Check sheet for the modelled part. Datum: model origin and axes. Units: mm. A direction names the side the tool comes from. Give positions to 0.01 mm unless a question says otherwise; leave off trailing zeros. Order: outer loops, then holes, each group sorted by start corner. A loop starts at its lowest first (then second) coordinate and runs counter-clockwise, first axis right, second up.
```python
from build123d import *

# Parameters (mm, degrees)
CROQUIS1_R              = 5.3
CROQUIS1_R_2            = 1.511434147
SALIENTE_EXTRUIR1_DEPTH = 3
CROQUIS3_R              = 1.8
CROQUIS3_R_2            = 5.3
SALIENTE_EXTRUIR2_DEPTH = 3


with BuildPart() as part:
    # Croquis1 → Saliente-Extruir1 (new body)
    with BuildSketch(Plane(origin=(0, 0, 0), x_dir=(1, 0, 0), z_dir=(0, 1, 0))):
        with BuildLine():
            Line((10.649291245, -23.45570863), (10.649291245, 1.133383189))
            ThreePointArc((10.649291245, 1.133383189), (-1.350708755, 19.76429137), (-13.350708755, 1.133383189))
            Line((-13.350708755, 1.133383189), (-13.350708755, -23.45570863))
            Line((-13.350708755, -23.45570863), (10.649291245, -23.45570863))
        make_face()
        with Locations((-1.350708755, 6.58429137)):
            Circle(CROQUIS1_R, mode=Mode.SUBTRACT)
        with Locations((6.073912448, 14.008912573)):
            Circle(CROQUIS1_R_2, mode=Mode.SUBTRACT)
        with Locations((6.073912448, -0.840329832)):
            Circle(CROQUIS1_R_2, mode=Mode.SUBTRACT)
        with Locations((-8.775329957, -0.840329832)):
            Circle(CROQUIS1_R_2, mode=Mode.SUBTRACT)
        with Locations((-8.775329957, 14.008912573)):
            Circle(CROQUIS1_R_2, mode=Mode.SUBTRACT)
    extrude(amount=SALIENTE_EXTRUIR1_DEPTH)

    # Croquis3 → Saliente-Extruir2 (add)
    with BuildSketch(Plane.XY.offset(23.45570863)):
        with BuildLine():
            Line((10.649291245, 3), (-13.350708755, 3))
            Line((-13.350708755, 3), (-13.350708755, -22.057235679))
            ThreePointArc((-13.350708755, -22.057235679), (-1.494791792, -40.779605827), (10.649291245, -22.242854272))
            Line((10.649291245, -22.242854272), (10.649291245, 3))
        make_face()
        with Locations((-8.817480498, -35.024621202)):
            Circle(CROQUIS3_R, mode=Mode.SUBTRACT)
        with Locations((-8.817480498, -20.175378798)):
            Circle(CROQUIS3_R, mode=Mode.SUBTRACT)
        with Locations((6.031761906, -20.175378798)):
            Circle(CROQUIS3_R, mode=Mode.SUBTRACT)
        with Locations((6.031761906, -35.024621202)):
            Circle(CROQUIS3_R, mode=Mode.SUBTRACT)
        with Locations((-1.392859296, -27.6)):
            Circle(CROQUIS3_R_2, mode=Mode.SUBTRACT)
    extrude(amount=SALIENTE_EXTRUIR2_DEPTH)


solid = part.part
```
Q1. Tool access check on faces 1 (the flat face through (-2, 0, 2)), 2 (the flat face through (-2, -19, 26.456)), 3 (the flat face through (10.649, 1, 18)). Record the directions out of +Z, -Z, +X, -X, +Y, -Y that give a thin tool (end or side, any length) a straight path to the whole face; none if there is none.
Q2. Sectioned sample at D-D, the plane z = -9. Record the cut outline in (x, y), plus the area to 3 significant figures.
Q3. Sectioned sample at C-C, the plane x = -9.25. Record the cut outline in (y, z).
Q4. Material ranges on line 1 (Y direction, x = 4.5, z = 20.5); line 2 (Z direction, x = 3.25, y = -35), recorded low to high.
Q5. Sectioned sample at A-A, the plane y = -27.6. Record the cut outline in (x, z), plus the area to 3 significant figures.
Q6. Sectioned sample at B-B, the plane x = -4.5. Record the cut outline in (y, z), plus the area to 3 significant figures.
Q7. Draft check along X on faces 4 (the flat face through (-13.351, 1, 19)), 5 (the flat face through (-2, -20, 23.456)), 6 (the cylindrical face through (1.5, 1.48, -11.05)). Enter one of: pulls with the +X half, pulls with the -X half, needs draft (parallel to the pull), parting line crosses it, or undercut.
Q8. Go/stop test with flat-tipped pins: P1, Ø8, axis at x = 5, y = -22.5, coming from the -Z side; P2, Ø13, axis at x = -0.5, z = -2.5, coming from the -Y side. Record where each tip stops, or that it passes through.
Filled in:
1. face 1: -Z, +X, -X, -Y
1. face 2: +Z, +X, -X, +Y, -Y
1. face 3: +Z, +X, +Y
2. outline: (-14.31, 0) - (-6.07, 0) - (-6.07, 3) - (-14.31, 3) - close; (3.37, 0) - (11.61, 0) - (11.61, 3) - (3.37, 3) - close
2. area: 49.4 mm2
3. outline: (-38.18, 23.46) - (-36.77, 23.46) - (-36.77, 26.46) - (-38.18, 26.46) - close; (-33.28, 23.46) - (-21.92, 23.46) - (-21.92, 26.46) - (-33.28, 26.46) - close; (-18.43, 23.46) - (0, 23.46) - (0, 2.28) - (3, 2.28) - (3, 26.46) - (-18.43, 26.46) - close; (0, -17.13) - (3, -17.13) - (3, -15.44) - (0, -15.44) - close; (0, -12.57) - (3, -12.57) - (3, -0.59) - (0, -0.59) - close
4. line 1: y = 0 to 3
4. line 2: z = 23.46 to 26.46
5. outline: (-14.57, 23.46) - (-6.69, 23.46) - (-6.69, 26.46) - (-14.57, 26.46) - close; (3.91, 23.46) - (11.79, 23.46) - (11.79, 26.46) - (3.91, 26.46) - close
5. area: 47.3 mm2
6. outline: (-40.41, 23.46) - (-31.89, 23.46) - (-31.89, 26.46) - (-40.41, 26.46) - close; (-23.31, 23.46) - (0, 23.46) - (0, -2.32) - (3, -2.32) - (3, 26.46) - (-23.31, 26.46) - close; (0, -19.38) - (3, -19.38) - (3, -10.85) - (0, -10.85) - close
6. area: 207 mm2
7. face 4: pulls with the -X half
7. face 5: needs draft
7. face 6: undercut
8. P1: stops at z = 23.46
8. P2: stops at y = 0
